Geometry: final body of the model. Coordinates: model frame, mm. Face numbers are marked on the shaded views. A direction names the side the tool comes from. Coordinates: 2 decimals unless noted, no trailing zeros. Order: outer loops, then holes, each group sorted by start corner. A loop starts at its lowest first (then second) coordinate and runs counter-clockwise, first axis right, second up. Notation, with made-up numbers: M 54,-4.75 L 99,-4.75 A14 ccw 99,17.25 Z; hole C 34.25,-8.5 d11. An arc over 180 degrees is marked long. Use CSV: the item, a comma, the result in double quotes. Start each with the question number.
Q1. Section query C-C, the plane y = 55.5. Output: boundary loops of the cut face in (x, z).
Q2. First-contact query: P1, Ø4, axis at x = 13, z = -1.5, coming from the -Y side; P2, Ø1.6, axis at x = -12, z = -6, coming from the +Y side; P3, Ø8, axis at y = 48, z = 4, coming from the +X side. Flat tips, straight axial feed; report the tip coordinate or a pass-through.
Q3. Mould query, pull axis Y, two halves, no side actions, for the marked faces 1, 2 and 3. Classes: +Y half, -Y half, draft (parallel to the pull), parting line (faces both ways), or undercut.
Q4. Section query A-A, the plane z = 6. State how many separate pieces and enclosed holes the cut face has, and give its area (3 significant figures).
Q5. Section query B-B, the plane x = 12. Output: boundary loops of the cut face in (y, z).
Q6. Access query for the marked faces 4 and 5. Directions: +Z, -Z, +X, -X, +Y, -Y. A direction counts if a zero-diameter tool reaches every point of the face in a straight line with its end or side. Return the directions, or none.
Q7. Ray query, probe 1 along X at (y, z) = (129.05, 6); probe 2 along Z at (x, y) = (-12, 128.7); probe 3 along Y at (x, z) = (-10.25, 5.25). Return the intervals inside material, ascending.
Q8. Section query D-D, the plane z = -1.25. Output: boundary loops of the cut face in (x, y), and give its area (3 significant figures).
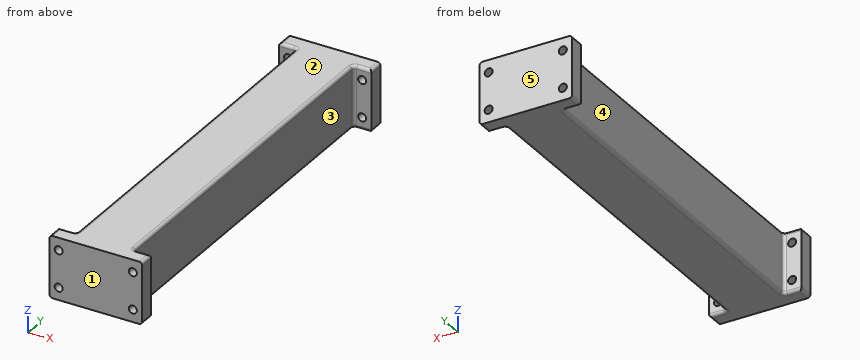
from build123d import *

# Parameters (mm, degrees)
SKETCH1_W           = 30
SKETCH1_H           = 20
SKETCH1_R           = 1.3
BOSS_EXTRUDE1_DEPTH = 5
SKETCH2_W           = 18.5
SKETCH2_H           = 20
BOSS_EXTRUDE2_DEPTH = 120
FILLET1_R           = 1


with BuildPart() as part:
    # Sketch1 → Boss-Extrude1 (new body)
    with BuildSketch(Plane(origin=(0, 0, 0), x_dir=(1, 0, 0), z_dir=(0, 1, 0))):
        Rectangle(SKETCH1_W, SKETCH1_H)
        with Locations((-12, 6)):
            Circle(SKETCH1_R, mode=Mode.SUBTRACT)
        with Locations((12, 6)):
            Circle(SKETCH1_R, mode=Mode.SUBTRACT)
        with Locations((12, -6)):
            Circle(SKETCH1_R, mode=Mode.SUBTRACT)
        with Locations((-12, -6)):
            Circle(SKETCH1_R, mode=Mode.SUBTRACT)
    boss_extrude1 = extrude(amount=BOSS_EXTRUDE1_DEPTH)

    # Sketch2 → Boss-Extrude2 (add)
    with BuildSketch(Plane(origin=(0, 5, 0), x_dir=(1, 0, 0), z_dir=(0, 1, 0))):
        Rectangle(SKETCH2_W, SKETCH2_H)
    extrude(amount=BOSS_EXTRUDE2_DEPTH)

    # Mirror1: Boss-Extrude1 across plane
    add(boss_extrude1.mirror(Plane.ZX.offset(65)))

    # Fillet1
    fillet1_edges = [part.edges().sort_by_distance(p)[0] for p in [
        (-12.125, 5, 10),
        (-12.125, 5, -10),
        (12.125, 5, 10),
        (9.25, 5, 0),
        (9.25, 65, 10),
        (9.25, 65, -10),
        (-9.25, 5, 0),
        (-9.25, 65, -10),
        (-9.25, 65, 10),
        (9.25, 125, 0),
        (-9.25, 125, 0),
        (15, 127.5, -10),
        (-12.125, 125, 10),
        (12.125, 125, 10),
        (15, 127.5, 10),
        (-15, 127.5, 10),
        (12.125, 125, -10),
        (-12.125, 125, -10),
        (-15, 127.5, -10),
        (15, 2.5, 10),
        (-15, 2.5, 10),
        (-15, 2.5, -10),
        (15, 2.5, -10),
        (12.125, 5, -10),
    ]]
    fillet(fillet1_edges, radius=FILLET1_R)


solid = part.part
Responses:
1,outline,"M -9.25,-9 A1 ccw -8.25,-10 L 8.25,-10 A1 ccw 9.25,-9 L 9.25,9 A1 ccw 8.25,10 L -8.25,10 A1 ccw -9.25,9 Z"
2,P1,"stops at y = 0"
2,P2,"passes through"
2,P3,"stops at x = 9.25"
3,face 1,"-Y half"
3,face 2,"draft"
3,face 3,"undercut"
4,separate pieces,"5"
4,enclosed holes,"0"
4,area,"2,470 mm²"
5,outline,"M 0,-10 L 4,-10 A1 ccw 5,-9 L 5,-7.3 L 0,-7.3 Z; M 0,-4.7 L 5,-4.7 L 5,4.7 L 0,4.7 Z; M 0,7.3 L 5,7.3 L 5,9 A1 ccw 4,10 L 0,10 Z; M 125,-9 A1 ccw 126,-10 L 130,-10 L 130,-7.3 L 125,-7.3 Z; M 125,-4.7 L 130,-4.7 L 130,4.7 L 125,4.7 Z; M 125,7.3 L 130,7.3 L 130,10 L 126,10 A1 ccw 125,9 Z"
6,face 4,"+Z, -Z, -X"
6,face 5,"+Z, -Z, +X, -X, +Y"
7,probe 1,"x = -15 to -13.3, -10.7 to 10.7, 13.3 to 15"
7,probe 2,"z = -10 to -7.3, -4.7 to 4.7, 7.3 to 10"
7,probe 3,"y = 0 to 5, 125 to 130"
8,outline,"M -15,0 L 15,0 L 15,5 L 10.25,5 A1 cw 9.25,6 L 9.25,124 A1 cw 10.25,125 L 15,125 L 15,130 L -15,130 L -15,125 L -10.25,125 A1 cw -9.25,124 L -9.25,6 A1 cw -10.25,5 L -15,5 Z"
8,area,"2,520 mm²"
